Autodesk Inventor part; units mm, degrees
ref_plane "Start plane" through (0, 0, 0) normal (0, 0, 1) x (1, 0, 0)
ref_plane "End plane" through (0, 0, 950) normal (0, 0, 1) x (1, 0, 0)
ref_plane "YZ Plane" through (0, 0, 0) normal (1, 0, 0) x (0, 1, 0)
ref_plane "Start plane" through (0, 0, 0) normal (0, 0, 1) x (1, 0, 0)
ref_plane "End plane" through (0, 0, 950) normal (0, 0, 1) x (1, 0, 0)
sketch "Sketch" plane through (0, 0, 0) normal (0, 0, 1) x (1, 0, 0)
  line L0 (-20, -14) -> (-20, 14)
  line L1 (-14, 20) -> (14, 20)
  line L2 (20, 14) -> (20, -14)
  line L3 (14, -20) -> (-14, -20)
  arc A0 (-20, -14) -> (-14, -20) centre (-14, -14) ccw
  arc A1 (-14, 20) -> (-20, 14) centre (-14, 14) ccw
  arc A2 (20, 14) -> (14, 20) centre (14, 14) ccw
  arc A3 (14, -20) -> (20, -14) centre (14, -14) ccw
  line L4 (-12, 16) -> (12, 16)
  line L5 (16, 12) -> (16, -12)
  line L6 (12, -16) -> (-12, -16)
  line L7 (-16, -12) -> (-16, 12)
  line L8 (0, 29.7397) -> (0, -29.7397) construction
  line L9 (-29.7397, 0) -> (29.7397, 0) construction
  arc A4 (-16, -12) -> (-12, -16) centre (-12, -12) ccw
  arc A5 (-12, 16) -> (-16, 12) centre (-12, 12) ccw
  arc A6 (16, 12) -> (12, 16) centre (12, 12) ccw
  arc A7 (12, -16) -> (16, -12) centre (12, -12) ccw
  dimension "d7" = 6
  dimension "d10" = 40
  dimension "d11" = 40
  dimension "d12" = 4
  dimension "d15" = 20
  dimension "d16" = 20
  dimension "d19" = 4
  dimension "d20" = 4
extrude "Body" add sketch "Sketch" along normal up to surface (950 mm away) from surface at 0
sketch "Sketch3" plane through (0, 0, 0) normal (0, 0, 1) x (1, 0, 0)
  line L0 (0, 0) -> (10, 0)
ref_plane "Work Plane3" through (0, 0, 0) normal (0, -1, 0) x (1, 0, 0)
sketch "Sketch4" plane through (0, 0, 0) normal (0, -1, 0) x (1, 0, 0)
  line L0 (-2, 0) -> (12, 0)
  line L1 (-2, 950) -> (12, 950)
  dimension "d18" = 950
sketch "Sketch5" plane through (0, -20, 0) normal (1, 0, 0) x (0, 1, 0)
  line L0 (20, 0) -> (20, 75)
  point P0 (20, 50)
  dimension "d21" = 75
  dimension "d22" = 25
hole "Hole1" at (0, 0, 50) at (0, 0, 75) direction (1, 0, 0) diameter 9 end through all
sketch "Sketch6" plane through (0, 0, 0) normal (1, 0, 0) x (0, 1, 0)
  circle A0 centre (25, 800) radius 15
  circle A1 centre (25, 800) radius 12.5
  point P0 (0, 0)
  dimension "d30" = 30
  dimension "d31" = 800
  dimension "d35" = 25
  dimension "d36" = 25
extrude "Extrusion2" cut sketch "Sketch6" against normal through all both and the other way through all contours A0 | A1
extrude "Extrusion3" add sketch "Sketch6" along normal mid plane 60
mirror "Mirror1" about plane through (0, 0, 0) normal (1, 0, 0) of "Hole1"
equation "\"d7\" = G_IR"
equation "\"d10\" = G_H"
equation "\"d11\" = G_W"
equation "\"d12\" = G_T"
equation "\"d15\" = 0.5 * d10"
equation "\"d16\" = 0.5 * d11"
equation "\"d19\" = G_T"
equation "\"d20\" = G_T"
equation "\"d3\" = G_L"
equation "\"G_W\" = 40"
equation "\"G_H\" = 40"
equation "\"G_T\" = 4"
equation "\"G_IR\" = 6"
equation "\"G_L\" = d18"
equation "\"G_OFFSET_START\" = 0"
equation "\"G_OFFSET_END\" = 0"
properties part number "EN 10210-2 - 40 x 40 x 4 - 950" material "Steel, Mild"
Design review of the part built by this model. Coordinates are the model's own, in mm. A direction names the side the tool comes from. Coordinates: 2 decimals unless noted, no trailing zeros. Loops run counter-clockwise (first coordinate to the right, second up) from the corner with the lowest first, then second, coordinate; pieces in that order, holes last. Notation, with made-up numbers: M 86,33 L 133,33 A34 cw 133,65 Z; hole C -22,-31 d4. An arc over 180 degrees is marked long. Answer as CSV lines item,"result".
Item 1: The part is to be moulded in two halves that separate along Y. For faces 6 (the face through (0, -20, 468)), 7 (the face through (20, 0, 468)), 8 (the face through (0, 16, 388)), say which applies: pulls with the +Y half, pulls with the -Y half, needs draft (parallel to the pull), parting line crosses it, or undercut.
Answer list:
face 6,"pulls with the -Y half"
face 7,"needs draft"
face 8,"undercut"
Item 2: Add section A-A on z = 282. State the section outline as (x, y) points.
Answer list:
outline,"M -20,-14 A6 ccw -14,-20 L 14,-20 A6 ccw 20,-14 L 20,14 A6 ccw 14,20 L -14,20 A6 ccw -20,14 Z; hole M -16,-12 A4 ccw -12,-16 L 12,-16 A4 ccw 16,-12 L 16,12 A4 ccw 12,16 L -12,16 A4 ccw -16,12 Z"
Item 3: For P1, Ø10.5, axis at y = 0, z = 75, coming from the +X side; P2, Ø3, axis at x = 22.5, z = 217.5, coming from the -Y side; P3, Ø22.5, axis at y = 0.5, z = 463.5, coming from the -X side; P4, Ø1, axis at x = 15, z = 373.5, coming from the -Y side, all flat-tipped, find the tip position at first contact; note any pin that passes through.
Answer list:
P1,"x = 20"
P2,"through"
P3,"x = -20"
P4,"y = -19.98"
Item 4: Machinability: for faces 1 (the face through (0, 16, 880)), 2 (the face through (0, 10, 800)), 3 (the face through (0, -16, 468)), 4 (the face through (-30, 21.6, 812.3)), 5 (the face through (-18, 0, 0)), which of the approach directions +Z, -Z, +X, -X, +Y, -Y give a long, thin tool a straight path to every point of the face, cutting with its end or side? Answer none if there is none.
Answer list:
face 1,"+Z"
face 2,"none"
face 3,"+Z, -Z"
face 4,"+Z, -Z, -X, +Y, -Y"
face 5,"-Z, +X, -X, +Y, -Y"
Item 5: For probe 1 along Y at (x, z) = (-12, 800); probe 2 along X at (y, z) = (-1.5, 399); probe 3 along X at (y, z) = (13, 568.5), list the stretches that pass through material, from the lowest coordinate up.
Answer list:
probe 1,"-20 to -16, 10 to 12.5, 37.5 to 40"
probe 2,"-20 to -16, 16 to 20"
probe 3,"-20 to -15.87, 15.87 to 20"
